Build history of the part. All positions in model axes, mm. A direction names the side the tool comes from. Give positions to 0.01 mm unless a question says otherwise; leave off trailing zeros. Loops run counter-clockwise (first coordinate to the right, second up) from the corner with the lowest first, then second, coordinate; pieces in that order, holes last. Notation, with made-up numbers: (50, 38) -> (98, 38) arc R8 cw to (98, 48) -> close; hole circle Ø10 at (55.25, 32). An arc over 180 degrees is marked (long way). Answer as a JSON object with one key per item and string values. Group by question number.
Q1. Band-saw the part on A-A, the plane x = 103. Write the cut outline in (y, z).
Q2. Two-plate mould, pull along X, no slides. Class faces 1 (the cylindrical face through (117.21, -50.59, 32.26)), 2 (the flat face through (36, 0, 0)), 3 (the flat face through (130.16, 18, -18)): pulls with the +X half, pulls with the -X half, needs draft (parallel to the pull), parting line crosses it, or undercut.
Q3. Wall check: probe 1 along X at (y, z) = (19, 30.5); probe 2 along X at (y, z) = (44, -27); probe 3 along Y at (x, z) = (118, 0.5). Give the ranges that are in metal, low to high. Write a range as from..to.
Q4. Band-saw the part on B-B, the plane x = 50. Write the cut outline in (y, z), plus the area to 3 significant figures.
Q5. Drop flat-ended pins along their axis: pin 1 (1 mm diameter, centred on x = 107, z = 38.5, fed in from -Y); pin 2 (5 mm diameter, centred on x = 100.5, z = -25, fed in from -Y); pin 3 (3 mm diameter, centred on x = 77.5, y = -2.5, fed in from +Z). Give the stop position or say it passes through.
Q6. Tool access for faces 4 (the flat face through (140, 5, 0)), 5 (the cylindrical face through (93.94, -15.02, 47.69)), 6 (the cylindrical face through (45.021, -16.855, -2.213)), 7 (the cylindrical face through (134.695, 21.477, -4.769)): list every direction of +Z, -Z, +X, -X, +Y, -Y with a clear straight run to the whole face (end or side of a thin tool).
from build123d import *

# Parameters (mm, degrees)
CUT_EXTRUDE1_DEPTH      = 4
CUT_EXTRUDE2_DEPTH      = 139.260282077
CUT_EXTRUDE2_DEPTH_BACK = 3
SKETCH3_R               = 8.5


with BuildPart() as part:
    # Sketch1 → Revolve1 (revolve)
    with BuildSketch(Plane.XY, mode=Mode.PRIVATE) as revolve1_sk:
        Polygon((0, 0), (0, 6), (33, 6), (33, 8.5), (43.5, 8.5), (43.5, 17), (46.5, 17), (46.5, 36.31855833), (53.568965517, 50), (66.568965517, 50), (66.568965517, 60), (73.751034483, 60), (73.751034483, 50), (113.568965517, 50), (113.568965517, 60), (120.751034483, 60), (120.751034483, 50), (127.16, 50), (127.16, 22), (130.16, 22), (130.16, 42), (132.16, 42), (132.16, 22), (137.16, 22), (137.16, 7), (142.16, 7), (142.16, 0), align=None)
    revolve(revolve1_sk.sketch.rotate(Axis((0, 0, 0), (1, 0, 0)), 90), axis=Axis((0, 0, 0), (1, 0, 0)))

    # Sketch2 → Cut-Extrude1 (cut)
    with BuildSketch(Plane(origin=(142.16, 0, 0), x_dir=(0, 0, -1), z_dir=(1, 0, 0))):
        with BuildLine():
            Line((-4.898979486, 5), (4.898979486, 5))
            ThreePointArc((4.898979486, 5), (0, 7), (-4.898979486, 5))
        make_face()
        with BuildLine():
            Line((-4.898979486, -5), (4.898979486, -5))
            ThreePointArc((4.898979486, -5), (0, -7), (-4.898979486, -5))
        make_face()
    extrude(amount=-CUT_EXTRUDE1_DEPTH, mode=Mode.SUBTRACT)

    # Sketch3 → Cut-Extrude2 (cut, two sides: drawn at the far end of the back side and taken through both)
    with BuildSketch(Plane.ZY.offset(-33).offset(-CUT_EXTRUDE2_DEPTH_BACK)):
        Circle(SKETCH3_R)
    extrude(amount=CUT_EXTRUDE2_DEPTH + CUT_EXTRUDE2_DEPTH_BACK, mode=Mode.SUBTRACT)


solid = part.part
Worked answers:
{
 "1": {"outline": "circle Ø100 at (0, 0)"},
 "2": {"face 1": "needs draft", "face 2": "pulls with the -X half", "face 3": "undercut"},
 "3": {"probe 1": "46.5..127.16, 130.16..132.16", "probe 2": "66.57..73.75, 113.57..120.75", "probe 3": "-60..60"},
 "4": {"outline": "circle Ø86.19 at (0, 0)", "area": "5,830 mm2"},
 "5": {"pin 1": "y = -32.5", "pin 2": "y = -44.65", "pin 3": "z = 49.99"},
 "6": {"face 4": "+Z, -Z, +X, +Y", "face 5": "none", "face 6": "-X", "face 7": "+X"}
}
